```python
from build123d import *

# Parameters (mm, degrees)
SKETCH_W             = 50
SKETCH_H             = 51
PAD_DEPTH            = 3
CHAMFER_SIZE         = 5
SKETCH001_W          = 50
SKETCH001_H          = 51
PAD001_DEPTH         = 3
CHAMFER001_SIZE      = 5
POCKET_DEPTH         = 207.576403
SKETCH003_R          = 1.5
SKETCH003_R_2        = 11
POCKET001_DEPTH      = 0.001
POCKET001_DEPTH_BACK = -51.001
PAD002_DEPTH         = 25
POCKET002_DEPTH      = 22


with BuildPart() as part:
    # Sketch → Pad (new body)
    with BuildSketch(Plane.XY):
        Rectangle(SKETCH_W, SKETCH_H)
    extrude(amount=PAD_DEPTH)

    # Chamfer
    chamfer_edges = [part.edges().sort_by_distance(p)[0] for p in [
        (25, -25.5, 1.5),
        (-25, -25.5, 1.5),
    ]]
    chamfer(chamfer_edges, length=CHAMFER_SIZE)

    # Sketch001 (on Face4 of Chamfer) → Pad001 (join)
    with BuildSketch(Plane(origin=(0, 25.5, 0), x_dir=(-1, 0, 0), z_dir=(0, 1, 0))):
        with Locations((0, 25.5)):
            Rectangle(SKETCH001_W, SKETCH001_H)
    extrude(amount=PAD001_DEPTH)

    # Chamfer001
    chamfer001_edges = [part.edges().sort_by_distance(p)[0] for p in [
        (-25, 27, 51),
        (25, 27, 51),
    ]]
    chamfer(chamfer001_edges, length=CHAMFER001_SIZE)

    # Sketch002 → Pocket (cut, through all)
    with BuildSketch(Plane.XZ):
        with BuildLine():
            ThreePointArc((-12.865, 39.85), (-15.015, 42), (-17.165, 39.85))
            Line((-17.165, 39.85), (-17.165, 10.15))
            ThreePointArc((-17.165, 10.15), (-15.015, 8), (-12.865, 10.15))
            Line((-12.865, 39.85), (-12.865, 10.15))
        make_face()
    pocket = extrude(amount=-POCKET_DEPTH, mode=Mode.SUBTRACT)

    # Mirrored: Pocket across Sketch002 V_Axis
    add(pocket.mirror(Plane(origin=(0, 0, 0), x_dir=(0, -1, 0), z_dir=(1, 0, 0))), mode=Mode.SUBTRACT)

    # Sketch003 → Pocket001 (cut, two sides)
    with BuildSketch(Plane.XY) as pocket001_sk:
        with Locations((-15.5, 11)):
            Circle(SKETCH003_R)
        with Locations((15.5, 11)):
            Circle(SKETCH003_R)
        with Locations((15.5, -20)):
            Circle(SKETCH003_R)
        with Locations((-15.5, -20)):
            Circle(SKETCH003_R)
        with Locations((0, -4.5)):
            Circle(SKETCH003_R_2)
    extrude(amount=-POCKET001_DEPTH, mode=Mode.SUBTRACT)
    extrude(pocket001_sk.sketch, amount=-POCKET001_DEPTH_BACK, mode=Mode.SUBTRACT)

    # Sketch004 → Pad002 (join, symmetric)
    with BuildSketch(Plane.YZ):
        Polygon((25.5, 22), (6.5, 3), (25.5, 3), align=None)
    extrude(amount=PAD002_DEPTH, both=True)

    # Sketch004 → Pocket002 (cut, symmetric)
    with BuildSketch(Plane.YZ):
        Polygon((25.5, 22), (6.5, 3), (25.5, 3), align=None)
    extrude(amount=POCKET002_DEPTH, both=True, mode=Mode.SUBTRACT)


solid = part.part
```
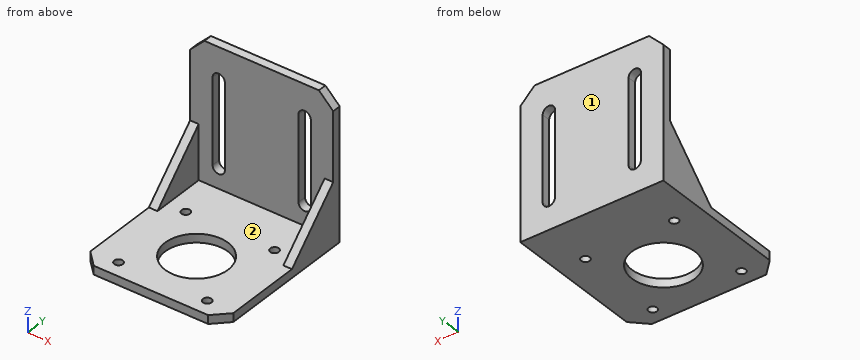
Check sheet for the modelled part. Datum: model origin and axes. Units: mm. Face numbers are marked on the shaded views. A direction names the side the tool comes from. Round coordinates to 2 decimals unless told otherwise and drop trailing zeros. Loops run counter-clockwise (first coordinate to the right, second up) from the corner with the lowest first, then second, coordinate; pieces in that order, holes last. Notation, with made-up numbers: M 23.5,48 L 72.5,48 A14 ccw 72.5,56 Z; hole C 17,41.5 d11. An arc over 180 degrees is marked long. Answer as a JSON object with one key per item and string values.
1. Section check A-A (x = 0). Record the boundary of the cut face in (y, z).
Reply:
{"outline": "M -25.5,0 L -15.5,0 L -15.5,3 L -25.5,3 Z; M 6.5,0 L 28.5,0 L 28.5,51 L 25.5,51 L 25.5,3 L 6.5,3 Z"}
2. Access from +Z, -Z, +X, -X, +Y, -Y to the whole of each face (thin tool, end or side, straight path). Record for the marked faces 1 and 2.
Reply:
{"face 1": "+Z, -Z, +X, -X, +Y", "face 2": "+Z, -Y"}
3. Section check C-C (y = -4.5). Record the boundary of the cut face in (x, z).
Reply:
{"outline": "M -25,0 L -11,0 L -11,3 L -25,3 Z; M 11,0 L 25,0 L 25,3 L 11,3 Z"}
4. Section check D-D (y = 14.5). Record the boundary of the cut face in (x, z).
Reply:
{"outline": "M -25,0 L 25,0 L 25,11 L 22,11 L 22,3 L -22,3 L -22,11 L -25,11 Z"}
5. Gauge pin test, flat ends, axial feed: P1, Ø2.5, axis at x = -15.5, y = -20, coming from the -Z side; P2, Ø5, axis at x = 15.5, y = -20, coming from the +Z side; P3, Ø4, axis at x = 14, z = 42.5, coming from the -Y side. Record the tip position at first contact, or that the pin passes through.
Reply:
{"P1": "passes through", "P2": "stops at z = 3", "P3": "stops at y = 25.5"}
6. Scan lines: line 1 (X direction, y = 11, z = 1); line 2 (Y direction, x = 15, z = 1); line 3 (Y direction, x = 0, z = 1.6). Record each from-to range of solid material in increasing order.
Reply:
{"line 1": "x = -25 to -17, -14 to 14, 17 to 25", "line 2": "y = -25.5 to -21.41, -18.59 to 9.59, 12.41 to 28.5", "line 3": "y = -25.5 to -15.5, 6.5 to 28.5"}
7. Section check B-B (z = 26.5). Record the boundary of the cut face in (x, y) (3 decimals).
Reply:
{"outline": "M -25,25.5 L -17.165,25.5 L -17.165,28.5 L -25,28.5 Z; M -12.865,25.5 L 12.865,25.5 L 12.865,28.5 L -12.865,28.5 Z; M 17.165,25.5 L 25,25.5 L 25,28.5 L 17.165,28.5 Z"}
